```python
from build123d import *

# Parameters (mm, degrees)
SKETCH_1_W          = 50
SKETCH_1_H          = 22
EXTRUDE_1_DEPTH     = 23
SKETCH_2_W          = 15.1
SKETCH_2_H          = 15.1
CUT_EXTRUDE_1_DEPTH = 77
SKETCH_3_R          = 2.25
CUT_EXTRUDE_2_DEPTH = 49
SKETCH_4_W          = 50
SKETCH_4_H          = 11.5
CUT_EXTRUDE_3_DEPTH = 49
FILLET_1_R          = 2
FILLET_2_R          = 2


with BuildPart() as part:
    # 草图1 → 凸台-拉伸1 (new body)
    with BuildSketch(Plane.XY):
        with Locations((25, -11)):
            Rectangle(SKETCH_1_W, SKETCH_1_H)
    extrude(amount=EXTRUDE_1_DEPTH)

    # 草图2 → 切除-拉伸1 (cut)
    with BuildSketch(Plane(origin=(50, 0, 0), x_dir=(0, 0, -1), z_dir=(1, 0, 0))):
        with Locations((-11.5, -11)):
            Rectangle(SKETCH_2_W, SKETCH_2_H)
    extrude(amount=-CUT_EXTRUDE_1_DEPTH, mode=Mode.SUBTRACT)

    # 草图3 → 切除-拉伸2 (cut)
    with BuildSketch(Plane(origin=(0, 0, 0), x_dir=(-1, 0, 0), z_dir=(0, 0, -1))):
        with Locations((-45, -11)):
            Circle(SKETCH_3_R)
        with Locations((-5, -11)):
            Circle(SKETCH_3_R)
    extrude(amount=-CUT_EXTRUDE_2_DEPTH, mode=Mode.SUBTRACT)

    # 草图4 → 切除-拉伸3 (cut)
    with BuildSketch(Plane.XZ.offset(22)):
        with Locations((25, 17.25)):
            Rectangle(SKETCH_4_W, SKETCH_4_H)
    extrude(amount=-CUT_EXTRUDE_3_DEPTH, mode=Mode.SUBTRACT)

    # 圆角1
    fillet_1_edges = [part.edges().sort_by_distance(p)[0] for p in [
        (25, 0, 0),
        (25, -22, 0),
    ]]
    fillet(fillet_1_edges, radius=FILLET_1_R)

    # 圆角2
    fillet_2_edges = [part.edges().sort_by_distance(p)[0] for p in [
        (0, 0, 6.75),
        (50, 0, 6.75),
        (50, -22, 6.75),
        (0, -22, 6.75),
        (0, -11, 0),
        (0, -21.414213562, 0.585786438),
        (0, -0.585786438, 0.585786438),
        (50, -11, 0),
        (50, -21.414213562, 0.585786438),
        (50, -0.585786438, 0.585786438),
    ]]
    fillet(fillet_2_edges, radius=FILLET_2_R)


solid = part.part
```
For this review, take the finished solid that the model builds, in its own axes (mm). A direction names the side the tool comes from. Give positions to 0.01 mm unless a question says otherwise; leave off trailing zeros. Loops run counter-clockwise (first coordinate to the right, second up) from the corner with the lowest first, then second, coordinate; pieces in that order, holes last. Notation, with made-up numbers: M 4,72 L 20,72 A21 cw 20,107 Z; hole C 70,79 d7. An arc over 180 degrees is marked long. One line per item, written item: value. Start each with the question number.
Q1. Add section C-C (x = 45). Give the boundary of the cut face in (y, z).
Q2. Clearance check with flat-ended pins moving along their axes: pin 1 Ø10 at (x, y) = (40.5, -8.5) entering from +Z; pin 2 Ø5 at (y, z) = (-14.5, 9) entering from -X. State where each tip first meets the part, or that it passes through.
Q3. Add section D-D (z = 1.5). Give the boundary of the cut face in (x, y).
Q4. Add section B-B (z = 5.25). Give the boundary of the cut face in (x, y).
Q5. Draft analysis for pull direction X (two halves, no side actions). For faces 3 (the face through (47.248, -10.901, 1.947)), 4 (the face through (25, -3.45, 8)), 5 (the face through (50, -11.1, 3.5)), state which applies: released by +X, released by -X, zero draft, split by the parting line, or undercut.
Q6. For L1, parallel to Y at x = 16, z = 8.75; L2, parallel to Y at x = 45, z = 1.85; L3, parallel to Z at x = 4.5, y = -15, list the stretches that pass through material, from the lowest coordinate up.
Q7. Machinability: for faces 1 (the face through (0.57, -0.6, 6.82)), 2 (the face through (25, -11, 3.95)), which of the approach directions +Z, -Z, +X, -X, +Y, -Y give a long, thin tool a straight path to every point of the face, cutting with its end or side? Answer none if there is none.
Q8. Add section A-A (y = -11). Give the boundary of the cut face in (x, z), and give its area (3 significant figures).
Reply:
1. outline: M -22,2 A2 ccw -20,0 L -13.25,0 L -13.25,3.95 L -18.55,3.95 L -18.55,11.5 L -22,11.5 Z; M -8.75,0 L -2,0 A2 ccw 0,2 L 0,11.5 L -3.45,11.5 L -3.45,3.95 L -8.75,3.95 Z
2. pin 1: z = 3.95
2. pin 2: through
3. outline: M 0.06,-20 A1.94 ccw 2,-21.94 L 48,-21.94 A1.94 ccw 49.94,-20 L 49.94,-2 A1.94 ccw 48,-0.06 L 2,-0.06 A1.94 ccw 0.06,-2 Z; hole C 5,-11 d4.5; hole C 45,-11 d4.5
4. outline: M 0,-20 A2 ccw 2,-22 L 48,-22 A2 ccw 50,-20 L 50,-18.55 L 0,-18.55 Z; M 0,-3.45 L 50,-3.45 L 50,-2 A2 ccw 48,0 L 2,0 A2 ccw 0,-2 Z
5. face 3: undercut
5. face 4: zero draft
5. face 5: released by +X
6. L1: -22 to -18.55, -3.45 to 0
6. L2: -21.99 to -13.25, -8.75 to -0.01
6. L3: 0 to 3.95
7. face 1: +Z, -Z, -X, +Y
7. face 2: +Z, +X, -X
8. outline: M 0,2 A2 ccw 2,0 L 2.75,0 L 2.75,3.95 L 0,3.95 Z; M 7.25,0 L 42.75,0 L 42.75,3.95 L 7.25,3.95 Z; M 47.25,0 L 48,0 A2 ccw 50,2 L 50,3.95 L 47.25,3.95 Z
8. area: 160 mm²
